Work out the finished part from the listing and answer in its coordinate system (mm). A direction names the side the tool comes from. Give positions to 0.01 mm unless a question says otherwise; leave off trailing zeros. Write each loop counter-clockwise with the first axis right and the second up, starting at its lowest first coordinate (ties: lowest second). Pieces come first, ordered by that corner, then holes. Notation, with made-up numbers: (66.25, -23) - (108.25, -23) arc R25 ccw to (108.25, -7) - close; hole circle Ø10 at (16, 30). An arc over 180 degrees is marked (long way). Write item = value, one per line.
from build123d import *

# Parameters (mm, degrees)
SKETCH1_W           = 19.9
SKETCH1_H           = 14
BOSS_EXTRUDE1_DEPTH = 9
SKETCH2_R           = 1.8
CUT_EXTRUDE1_DEPTH  = 20.390783893
CUT_EXTRUDE2_DEPTH  = 7.5


with BuildPart() as part:
    # Sketch1 → Boss-Extrude1 (new body)
    with BuildSketch(Plane.XY):
        with Locations((0, 7)):
            Rectangle(SKETCH1_W, SKETCH1_H)
    extrude(amount=BOSS_EXTRUDE1_DEPTH)

    # Sketch2 → Cut-Extrude1 (cut, through all)
    with BuildSketch(Plane(origin=(0, 14, 0), x_dir=(1, 0, 0), z_dir=(0, 1, 0))):
        with Locations(Location((0, -4.5, 0), (0, 0, 270))):
            Circle(SKETCH2_R)
    extrude(amount=-CUT_EXTRUDE1_DEPTH, mode=Mode.SUBTRACT)

    # Sketch3 → Cut-Extrude2 (cut)
    with BuildSketch(Plane.XY.offset(9)):
        Polygon((6, 14), (6, 0), (6.7, 0), (6.7, 0.2), (7.6, 1.1), (6.7, 2), (6.7, 2.2), (7.6, 3.1), (6.7, 4), (6.7, 4.2), (7.6, 5.1), (6.7, 6), (6.7, 6.2), (7.6, 7.1), (6.7, 8), (6.7, 8.2), (7.6, 9.1), (6.7, 10), (6.7, 10.2), (7.6, 11.1), (6.7, 12), (6.7, 12.2), (7.6, 13.1), (6.7, 14), align=None)
        Polygon((-6.7, 0.2), (-6.7, 0), (-6, 0), (-6, 14), (-6.7, 14), (-7.6, 13.1), (-6.7, 12.2), (-6.7, 12), (-7.6, 11.1), (-6.7, 10.2), (-6.7, 10), (-7.6, 9.1), (-6.7, 8.2), (-6.7, 8), (-7.6, 7.1), (-6.7, 6.2), (-6.7, 6), (-7.6, 5.1), (-6.7, 4.2), (-6.7, 4), (-7.6, 3.1), (-6.7, 2.2), (-6.7, 2), (-7.6, 1.1), align=None)
    extrude(amount=-CUT_EXTRUDE2_DEPTH, mode=Mode.SUBTRACT)


solid = part.part
1. Given pin 1 (0.8 mm diameter, centred on x = -6.5, y = 9.5, fed in from +Z), flat-ended and moving along its own axis, determine where the tip first touches the part or whether it passes through.
Solution:
pin_1 = 1.5
2. Find section B-B, the plane z = 4.5. Give the number of separate pieces and of enclosed holes in the cut face, then the cut area to 3 significant figures.
Solution:
separate_pieces = 4
enclosed_holes = 0
area = 197 mm^2
3. A tool of negligible diameter and unlimited length cuts with its end or side. For faces 4 (the flat face through (7.2, 5.5, 5.3)), 5 (the flat face through (9, 7, 9)), from which of +Z, -Z, +X, -X, +Y, -Y can it reach the whole face along a straight path? Write none if from no direction.
Solution:
face_4 = +Z
face_5 = +Z, +X, -X, +Y, -Y
4. Find section A-A, the plane x = 0. Give the vertices of the cut face in (y, z).
Solution:
outline = (0, 0) - (14, 0) - (14, 2.7) - (0, 2.7) - close; (0, 6.3) - (14, 6.3) - (14, 9) - (0, 9) - close
5. Straight lines are drawn through the part: line 1 (X direction, y = 3, z = 4.5); line 2 (X direction, y = 10.75, z = 4.5); line 3 (X direction, y = 11, z = 8.25). For each, find the intervals that lie inside material, in ascending order.
Solution:
line_1 = -9.95 to -7.5, -6 to -1.8, 1.8 to 6, 7.5 to 9.95
line_2 = -9.95 to -7.25, -6 to -1.8, 1.8 to 6, 7.25 to 9.95
line_3 = -9.95 to -7.5, -6 to 6, 7.5 to 9.95
6. For a pull along Y with two mould halves and no side action, classify faces 1 (the flat face through (-2, 14, 4)), 2 (the flat face through (-7.1, 5.6, 5.3)), 3 (the flat face through (-6, 7, 5)) as pulls with the +Y half, pulls with the -Y half, needs draft (parallel to the pull), parting line crosses it, or undercut.
Solution:
face_1 = pulls with the +Y half
face_2 = undercut
face_3 = needs draft
